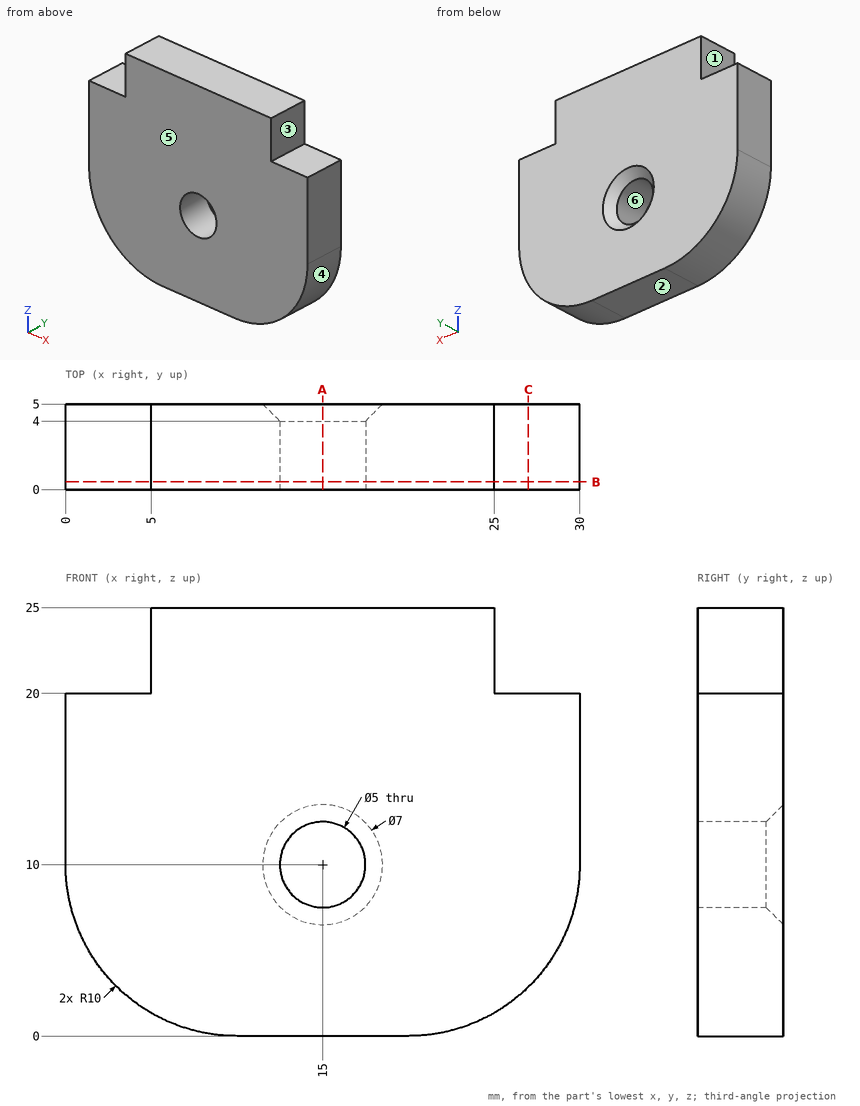
Geometry check sheet. Reference: drawing and pictorial views, mm from the part's lowest x, y, z. A direction names the side the tool comes from. Give positions to 0.01 mm unless a question says otherwise; leave off trailing zeros. Write each loop counter-clockwise with the first axis right and the second up, starting at its lowest first coordinate (ties: lowest second). Pieces come first, ordered by that corner, then holes. Notation, with made-up numbers: (-15.75, 32.25) - (36.25, 32.25) arc R22 ccw to (36.25, 42.25) - close; hole circle Ø6 at (-28.75, 76). An arc over 180 degrees is marked (long way). Put each result on its own line as item: value.
Q1. Scan lines: probe 1 along X at (y, z) = (1.45, 10); probe 2 along Z at (x, y) = (15, 0.95); probe 3 along Z at (x, y) = (28, 1.55). Record each from-to range of solid material in increasing order. Write a range as from..to.
Result:
probe 1: 0..12.5, 17.5..30
probe 2: 0..7.5, 12.5..25
probe 3: 4..20
Q2. Section check A-A on x = 15. Record the cut outline in (y, z).
Result:
outline: (0, 0) - (5, 0) - (5, 6.5) - (4, 7.5) - (0, 7.5) - close; (0, 12.5) - (4, 12.5) - (5, 13.5) - (5, 25) - (0, 25) - close
Q3. Section check C-C on x = 27. Record the cut outline in (y, z), and give its area (3 significant figures).
Result:
outline: (0, 2.86) - (5, 2.86) - (5, 20) - (0, 20) - close
area: 85.7 mm2
Q4. Mould release check, pull along X, two halves, no side actions. Record for the marked faces 4, 5 and 6: released by +X, released by -X, zero draft, split by the parting line, or undercut.
Result:
face 4: released by +X
face 5: zero draft
face 6: undercut
Q5. Set-up check for the marked faces 1, 2 and 3: record each of +Z, -Z, +X, -X, +Y, -Y from which the full face is reachable in a straight line by a thin tool's end or side.
Result:
face 1: +Z, -X, +Y, -Y
face 2: -Z, +X, -X, +Y, -Y
face 3: +Z, +X, +Y, -Y
Q6. Section check B-B on y = 0.45. Record the cut outline in (x, z), and give its area (3 significant figures).
Result:
outline: (0, 10) arc R10 ccw to (10, 0) - (20, 0) arc R10 ccw to (30, 10) - (30, 20) - (25, 20) - (25, 25) - (5, 25) - (5, 20) - (0, 20) - close; hole circle Ø5 at (15, 10)
area: 637 mm2
Q7. Depth check by flat-ended pin: P1, Ø6.5, axis at x = 15, z = 10, coming from the +Y side; P2, Ø1.5, axis at x = 2.5, y = 1.5, coming from the +Z side; P3, Ø1.5, axis at y = 2.5, z = 23.5, coming from the -X side. Enter the tip coordinate at first touch or a pass-through.
Result:
P1: y = 4.75
P2: z = 20
P3: x = 5
